The model under review builds one solid part; all positions refer to its coordinate system, in mm. A direction names the side the tool comes from. Give positions to 0.01 mm unless a question says otherwise; leave off trailing zeros. Order: outer loops, then holes, each group sorted by start corner. A loop starts at its lowest first (then second) coordinate and runs counter-clockwise, first axis right, second up. Notation, with made-up numbers: (-5.5, 17) - (19.5, 17) arc R21 cw to (19.5, 50) - close; hole circle Ø5 at (75, 3). An arc over 180 degrees is marked (long way). Use CSV: the item, a comma, the result in double quotes. Start each with the question number.
1. Take a section at B-B, the plane y = 0. State the section outline as (x, z) points, then the cut area to 3 significant figures.
2. For pin 1 (8 mm diameter, centred on x = 12.5, y = -21.65, fed in from +Z); pin 2 (12 mm diameter, centred on x = -30, y = -7.5, fed in from +Z); pin 3 (3 mm diameter, centred on x = -18, z = 25, fed in from +Y); pin 4 (14.5 mm diameter, centred on x = 14.5, y = 20.5, fed in from +Z), all flat-tipped, find the tip position at first contact; note any pin that passes through.
3. To check wall thickness, follow line 1 (Y direction, x = 0, z = 19.5); line 2 (X direction, y = -18, z = 7); line 3 (Y direction, x = -12.5, z = 6.9). State the ranges of each line that lie inside material, in increasing order. Write a range as [from, to].
4. Take a section at D-D, the plane z = 20. State the section outline as (x, y) points.
5. Take a section at A-A, the plane x = 25. State the section outline as (y, z) points, then the cut area to 3 significant figures.
6. Draft analysis for pull direction Y (two halves, no side actions). For faces 3 (the cylindrical face through (-4.88, -37.18, 16.76)), 4 (the cylindrical face through (-31.494, 0.286, 6.028)), 5 (the flat face through (-31, 17, 34)), state which applies: released by +Y, released by -Y, zero draft, split by the parting line, or undercut.
7. Take a section at C-C, the plane x = 12.5. State the section outline as (y, z) points, then the cut area to 3 significant figures.
8. Machinability: for faces 1 (the cylindrical face through (22.5, 0.1, 2)), 2 (the flat face through (25, -3, 4)), which of the approach directions +Z, -Z, +X, -X, +Y, -Y give a long, thin tool a straight path to every point of the face, cutting with its end or side? Answer none if there is none.
Autodesk Inventor part; units mm, degrees
ref_plane "YZ Plane" through (0, 0, 0) normal (1, 0, 0) x (0, 1, 0)
ref_plane "XZ Plane" through (0, 0, 0) normal (0, 1, 0) x (-1, 0, 0)
ref_plane "XY Plane" through (0, 0, 0) normal (0, 0, 1) x (1, 0, 0)
sketch "Sketch1" plane through (0, 0, 0) normal (0, 0, 1) x (1, 0, 0)
  circle A0 centre (0, 0) radius 37.5
  dimension "d0" = 75
extrude "Extrusion1" add sketch "Sketch1" along normal blind 34
sketch "Sketch2" plane through (0, 0, 34) normal (0, 0, 1) x (1, 0, 0)
  circle A0 centre (0, 0) radius 37.5
  circle A1 centre (0, 0) radius 35
  dimension "d105" = 70
extrude "Extrusion2" cut sketch "Sketch2" against normal blind 26 contours A1
sketch "Sketch3" plane through (0, 0, 8) normal (0, 0, 1) x (1, 0, 0)
  circle A0 centre (0, 0) radius 11
  dimension "d6" = 22
extrude "Extrusion3" cut sketch "Sketch3" against normal through all
sketch "Sketch4" plane through (0, 0, 8) normal (0, 0, 1) x (1, 0, 0)
  circle A0 centre (25, 0) radius 6.5
  circle A1 centre (12.5, 21.6506) radius 6.5
  circle A2 centre (-12.5, 21.6506) radius 6.5
  circle A3 centre (-25, 0) radius 6.5
  circle A4 centre (-12.5, -21.6506) radius 6.5
  circle A5 centre (12.5, -21.6506) radius 6.5
  point P0 (0, 0)
  dimension "d9" = 13
  dimension "d10" = 25
  dimension "d13" = 360
extrude "Extrusion4" cut sketch "Sketch4" against normal blind 4
sketch "Sketch5" plane through (0, 0, 8) normal (0, 0, 1) x (1, 0, 0)
  circle A0 centre (0, 0) radius 11 construction
  circle A1 centre (25, 0) radius 2.5
  circle A2 centre (12.5, 21.6506) radius 2.5
  circle A3 centre (-12.5, 21.6506) radius 2.5
  circle A4 centre (-25, 0) radius 2.5
  circle A5 centre (-12.5, -21.6506) radius 2.5
  circle A6 centre (12.5, -21.6506) radius 2.5
  dimension "d99" = 5
  dimension "d100" = 25
  dimension "d103" = 360
extrude "Extrusion5" cut sketch "Sketch5" against normal through all
sketch "Sketch6" plane through (0, 0, 8) normal (0, 0, 1) x (1, 0, 0)
  circle A0 centre (0, 20) radius 1.5
  circle A1 centre (-17.3205, 10) radius 1.5
  circle A2 centre (-17.3205, -10) radius 1.5
  circle A3 centre (0, -20) radius 1.5
  circle A4 centre (17.3205, -10) radius 1.5
  circle A5 centre (17.3205, 10) radius 1.5
  point P0 (0, 0)
  dimension "d24" = 3
  dimension "d25" = 20
  dimension "d28" = 360
extrude "Extrusion6" cut sketch "Sketch6" against normal through all
properties part number "Base" material "ABS Plastic"
Determined:
1,outline,"(-37.5, 0) - (-27.5, 0) - (-27.5, 4) - (-31.5, 4) - (-31.5, 8) - (-35, 8) - (-35, 34) - (-37.5, 34) - close; (-22.5, 0) - (-11, 0) - (-11, 8) - (-18.5, 8) - (-18.5, 4) - (-22.5, 4) - close; (11, 0) - (22.5, 0) - (22.5, 4) - (18.5, 4) - (18.5, 8) - (11, 8) - close; (27.5, 0) - (37.5, 0) - (37.5, 34) - (35, 34) - (35, 8) - (31.5, 8) - (31.5, 4) - (27.5, 4) - close"
1,area,"410 mm²"
2,pin 1,"stops at z = 4"
2,pin 2,"stops at z = 34"
2,pin 3,"stops at y = 33.67"
2,pin 4,"stops at z = 8"
3,line 1,"y = [-37.5, -35], [35, 37.5]"
3,line 2,"x = [-32.9, -17.88], [-7.12, 7.12], [17.88, 32.9]"
3,line 3,"y = [-35.36, -28.15], [-15.15, 15.15], [28.15, 35.36]"
4,outline,"circle Ø75 at (0, 0); hole circle Ø70 at (0, 0)"
5,outline,"(-27.95, 0) - (-2.5, 0) - (-2.5, 4) - (-6.5, 4) - (-6.5, 8) - (-24.49, 8) - (-24.49, 34) - (-27.95, 34) - close; (2.5, 0) - (27.95, 0) - (27.95, 34) - (24.49, 34) - (24.49, 8) - (6.5, 8) - (6.5, 4) - (2.5, 4) - close"
5,area,"555 mm²"
6,face 3,"split by the parting line"
6,face 4,"undercut"
6,face 5,"zero draft"
7,outline,"(-35.36, 0) - (-24.15, 0) - (-24.15, 4) - (-28.15, 4) - (-28.15, 8) - (-32.69, 8) - (-32.69, 34) - (-35.36, 34) - close; (-19.15, 0) - (19.15, 0) - (19.15, 4) - (15.15, 4) - (15.15, 8) - (-15.15, 8) - (-15.15, 4) - (-19.15, 4) - close; (24.15, 0) - (35.36, 0) - (35.36, 34) - (32.69, 34) - (32.69, 8) - (28.15, 8) - (28.15, 4) - (24.15, 4) - close"
7,area,"560 mm²"
8,face 1,"+Z, -Z"
8,face 2,"+Z"
